```python
from build123d import *

# Parameters (mm, degrees)
SKETCH_W    = 9
SKETCH_H    = 11
PAD_DEPTH   = 3
FILLET_R    = 1
FILLET001_R = 2.5


with BuildPart() as part:
    # Sketch → Pad (new body)
    with BuildSketch(Plane.XY):
        Polygon((39.740207, 35.73141), (39.740207, -4.26859), (36.490207, -4.26859), (36.490207, -7.26859), (26.590207, -7.26859), (26.590207, -4.26859), (23.340207, -4.26859), (23.340207, 35.73141), (26.590207, 35.73141), (26.590207, 38.73141), (36.490207, 38.73141), (36.490207, 35.73141), align=None)
        with Locations((32.540207, 11.73141)):
            Rectangle(SKETCH_W, SKETCH_H, mode=Mode.SUBTRACT)
    extrude(amount=PAD_DEPTH)

    # Fillet
    fillet_edges = [part.edges().sort_by_distance(p)[0] for p in [
        (36.490207, -7.26859, 1.5),
        (26.590207, -7.26859, 1.5),
        (36.490207, 38.73141, 1.5),
        (26.590207, 38.73141, 1.5),
    ]]
    fillet(fillet_edges, radius=FILLET_R)

    # Fillet001
    fillet001_edges = [part.edges().sort_by_distance(p)[0] for p in [
        (39.740207, -4.26859, 1.5),
        (39.740207, 35.73141, 1.5),
        (23.340207, -4.26859, 1.5),
        (23.340207, 35.73141, 1.5),
    ]]
    fillet(fillet001_edges, radius=FILLET001_R)


with BuildPart() as part_1:
    # Fillet001 placement: moved
    add(part.part.moved(Location((200, 100, 0))))


solid = part_1.part
```
Source: CAD feature listing. Evaluate the final solid. Frame: model axes, mm. A direction names the side the tool comes from. Give positions to 0.01 mm unless a question says otherwise; leave off trailing zeros. Write each loop counter-clockwise with the first axis right and the second up, starting at its lowest first coordinate (ties: lowest second). Pieces come first, ordered by that corner, then holes.
1. Section query B-B (z = 0.9). Return the cut outline in (x, y), then the cut area to 3 significant figures.
2. Section query C-C (x = 238.5). Return the cut outline in (y, z).
3. Section query D-D (x = 225). Return the cut outline in (y, z).
4. Section query A-A (x = 233.5). Return the cut outline in (y, z), then the cut area to 3 significant figures.
5. Material intervals for line 1 along X through (y, z) = (115, 2); line 2 along Y through (x, z) = (230, 0.1); line 3 along X through (y, z) = (136.5, 2.9), sorted ascending.
6. Access query for faces 4 (the face through (236.49, 137, 1)), 5 (the face through (226.59, 137, 1)), 6 (the face through (226.59, 95, 1)), 7 (the face through (232, 106.231, 1)), 8 (the face through (236.49, 95, 1)). Directions: +Z, -Z, +X, -X, +Y, -Y. A direction counts if a zero-diameter tool reaches every point of the face in a straight line with its end or side. Return the directions, or none.
7. Pull-direction query (Y, two-part tool) for faces 1 (the face through (236.205, 138.431, 1.521)), 2 (the face through (224.053, 96.483, 1.521)), 3 (the face through (237.04, 112, 1)); classes: +Y half, -Y half, draft (parallel to the pull), parting line (faces both ways), or undercut.
8. First-contact query: pin 1 (1 mm diameter, centred on y = 137, z = 2, fed in from +X); pin 2 (0.8 mm diameter, centred on x = 237, z = 2, fed in from +Y); pin 3 (6 mm diameter, centred on x = 238, y = 124.5, fed in from -Z); pin 4 (1.6 mm diameter, centred on y = 137, z = 1.5, fed in from -X). Flat tips, straight axial feed; report the tip coordinate or a pass-through.
Output values:
1. outline: (223.34, 98.23) arc R2.5 ccw to (225.84, 95.73) - (226.59, 95.73) - (226.59, 93.73) arc R1 ccw to (227.59, 92.73) - (235.49, 92.73) arc R1 ccw to (236.49, 93.73) - (236.49, 95.73) - (237.24, 95.73) arc R2.5 ccw to (239.74, 98.23) - (239.74, 133.23) arc R2.5 ccw to (237.24, 135.73) - (236.49, 135.73) - (236.49, 137.73) arc R1 ccw to (235.49, 138.73) - (227.59, 138.73) arc R1 ccw to (226.59, 137.73) - (226.59, 135.73) - (225.84, 135.73) arc R2.5 ccw to (223.34, 133.23) - close; hole (228.04, 106.23) - (237.04, 106.23) - (237.04, 117.23) - (228.04, 117.23) - close
1. area: 610 mm2
2. outline: (96.07, 0) - (135.39, 0) - (135.39, 3) - (96.07, 3) - close
3. outline: (95.88, 0) - (135.59, 0) - (135.59, 3) - (95.88, 3) - close
4. outline: (92.73, 0) - (106.23, 0) - (106.23, 3) - (92.73, 3) - close; (117.23, 0) - (138.73, 0) - (138.73, 3) - (117.23, 3) - close
4. area: 105 mm2
5. line 1: x = 223.34 to 228.04, 237.04 to 239.74
5. line 2: y = 92.73 to 106.23, 117.23 to 138.73
5. line 3: x = 226.59 to 236.49
6. face 4: +Z, -Z, +X, +Y
6. face 5: +Z, -Z, -X, +Y
6. face 6: +Z, -Z, -X, -Y
6. face 7: +Z, -Z
6. face 8: +Z, -Z, +X, -Y
7. face 1: +Y half
7. face 2: -Y half
7. face 3: undercut
8. pin 1: stops at x = 236.49
8. pin 2: stops at y = 135.73
8. pin 3: stops at z = 0
8. pin 4: stops at x = 226.59
